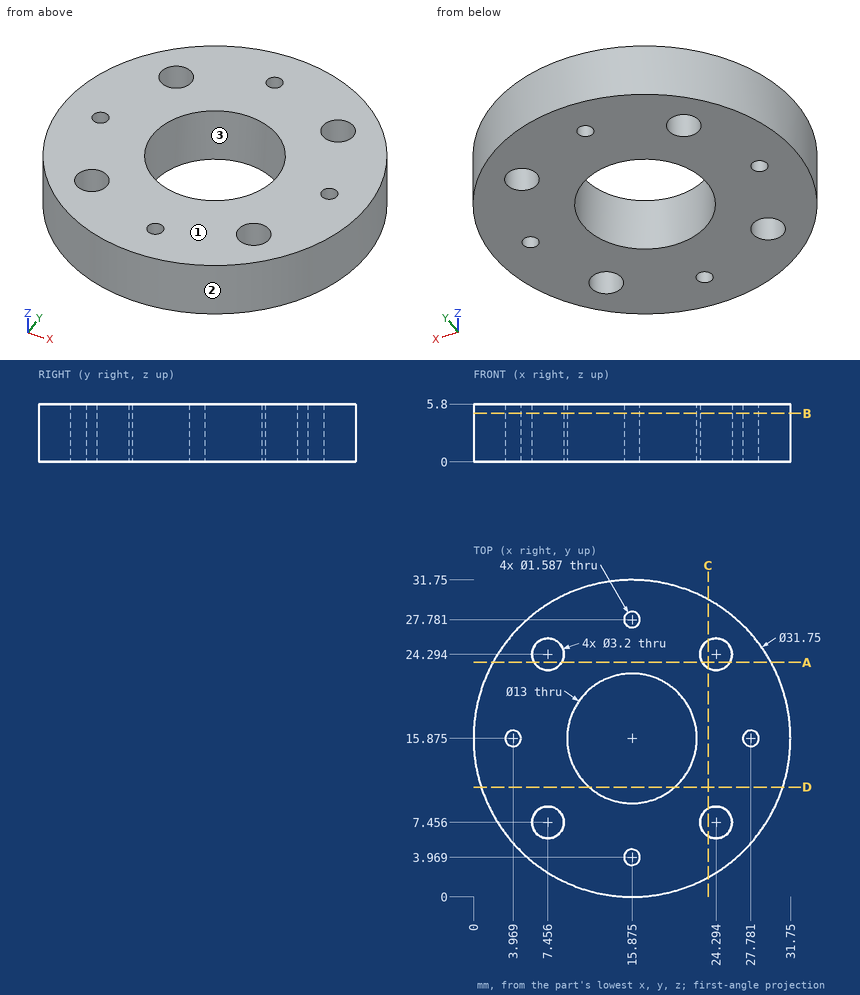
Could you check a few things on this drawing? It's one solid part, dimensions in mm from its lowest x, y, z. Round coordinates to 2 decimals unless told otherwise and drop trailing zeros. Loops run counter-clockwise (first coordinate to the right, second up) from the corner with the lowest first, then second, coordinate; pieces in that order, holes last.
Q1. For P1, Ø3, axis at x = 8.5, z = 3, coming from the +Y side; P2, Ø1.4, axis at x = 15.88, y = 3.97, coming from the -Z side; P3, Ø3, axis at y = 10, z = 2, coming from the +X side (1 decimal); P4, Ø1.5, axis at y = 28, z = 0.5, coming from the +X side, each with a flat end and sliding along its axis, tell me the tip position at first contact or that it passes through.
Q2. Please list where these lines run through material, in increasing order: L1, parallel to Y at x = 24.5, z = 0.6; L2, parallel to X at y = 16.5, z = 4 (1 decimal); L3, parallel to Y at x = 7.5, z = 2.6 (1 decimal).
Q3. I want a section at B-B (z = 4.85). Give the number of separate pieces and of enclosed holes in the cut face, and give its area (3 significant figures).
Q4. I want a section at D-D (y = 11). Write out the boundary of the cut face in (x, z) (1 decimal).
Q5. Thinking about a two-plate mould opening in Y: for the marked faces 1, 2 and 3, which applies, pulls with the +Y half, pulls with the -Y half, needs draft (parallel to the pull), parting line crosses it, or undercut?
Q6. I want a section at A-A (y = 23.5). Write out the boundary of the cut face in (x, z) (1 decimal), and give its area (3 significant figures).
Answer below:
1. P1: stops at y = 30.62
1. P2: passes through
1. P3: stops at x = 31.1
1. P4: stops at x = 26.95
2. L1: y = 2.55 to 5.87, 9.04 to 22.71, 25.88 to 29.2
2. L2: x = 0 to 3.5, 4.5 to 9.4, 22.3 to 27.3, 28.3 to 31.7
2. L3: y = 2.4 to 5.9, 9.1 to 22.7, 25.9 to 29.4
3. separate pieces: 1
3. enclosed holes: 9
3. area: 619 mm2
4. outline: (0.8, 0) - (11.6, 0) - (11.6, 5.8) - (0.8, 5.8) - close; (20.2, 0) - (31, 0) - (31, 5.8) - (20.2, 5.8) - close
5. face 1: needs draft
5. face 2: parting line crosses it
5. face 3: undercut
6. outline: (2, 0) - (6.1, 0) - (6.1, 5.8) - (2, 5.8) - close; (8.8, 0) - (22.9, 0) - (22.9, 5.8) - (8.8, 5.8) - close; (25.7, 0) - (29.8, 0) - (29.8, 5.8) - (25.7, 5.8) - close
6. area: 129 mm2
